Source: CAD feature listing. Evaluate the final solid. Frame: model axes, mm. Face numbers are marked on the shaded views. A direction names the side the tool comes from. Round coordinates to 2 decimals unless told otherwise and drop trailing zeros. Order: outer loops, then holes, each group sorted by start corner. A loop starts at its lowest first (then second) coordinate and runs counter-clockwise, first axis right, second up. Notation, with made-up numbers: (72, 41) -> (79, 41) arc R27 cw to (79, 59) -> close; hole circle Ø10 at (-37.75, 43.25). An arc over 180 degrees is marked (long way). Write item = value, one per line. Start each with the question number.
(1) Contact query for flat-ended pins moving along their axis: pin 1 Ø10.5 at (x, z) = (4, 6) entering from -Y; pin 2 Ø12 at (x, z) = (-2, -10) entering from +Y; pin 3 Ø5 at (y, z) = (-12, -2) entering from +X. Output: stop coordinate, or through.
(2) Cut plane C-C on z = -19. Return the cut outline in (x, y).
(3) Cut plane A-A on y = 0. Return the cut outline in (x, z), then the cut area to 3 significant figures.
(4) Draft query along Z for the marked faces 1, 2, 3 and 4. Return one class per face: released by +Z, released by -Z, zero draft, split by the parting line, or undercut.
(5) Cut plane D-D on x = 20.5. Return the cut outline in (y, z).
(6) Ray query, line 1 (Y direction, x = -0.5, z = -26.5); line 2 (X direction, y = 0, z = -26). Return the intervals inside material, ascending.
(7) Reachability of the marked faces 5, 6, 7, 8 and 9 from +Z, -Z, +X, -X, +Y, -Y: full face, straight path, thin tool, end or side. Return the list, or none.
from build123d import *

# Parameters (mm, degrees)
F2_W          = 60
F2_H          = 60
F3_DEPTH      = 30
F3_DEPTH_BACK = 30
F9_R          = 22.5
F10_DEPTH     = 12.5
F6_R          = 22.5
F11_DEPTH     = 12.5
F5_R          = 22.5
F12_DEPTH     = 12.5
F8_R          = 22.5
F13_DEPTH     = 12.5
F7_R          = 22.5
F14_DEPTH     = 12.5
F4_R          = 22.5
F15_DEPTH     = 12.5


with BuildPart() as f3:
    # F2 (on Top) → F3 (new body, two sides)
    with BuildSketch(Plane.XY) as f3_sk:
        Rectangle(F2_W, F2_H)
    extrude(amount=F3_DEPTH)
    extrude(f3_sk.sketch, amount=-F3_DEPTH_BACK)

    # F9 (on face) → F10 (cut)
    with BuildSketch(Plane(origin=(0, 0, -30), x_dir=(1, 0, 0), z_dir=(0, 0, -1))):
        Circle(F9_R)
    extrude(amount=-F10_DEPTH, mode=Mode.SUBTRACT)

    # F6 (on face) → F11 (cut)
    with BuildSketch(Plane(origin=(-30, 0, 0), x_dir=(0, -1, 0), z_dir=(-1, 0, 0))):
        Circle(F6_R)
    extrude(amount=-F11_DEPTH, mode=Mode.SUBTRACT)

    # F5 (on face) → F12 (cut)
    with BuildSketch(Plane.XZ.offset(30)):
        Circle(F5_R)
    extrude(amount=-F12_DEPTH, mode=Mode.SUBTRACT)

    # F8 (on face) → F13 (cut)
    with BuildSketch(Plane.YZ.offset(30)):
        Circle(F8_R)
    extrude(amount=-F13_DEPTH, mode=Mode.SUBTRACT)

    # F7 (on face) → F14 (cut)
    with BuildSketch(Plane(origin=(0, 30, 0), x_dir=(-1, 0, 0), z_dir=(0, 1, 0))):
        Circle(F7_R)
    extrude(amount=-F14_DEPTH, mode=Mode.SUBTRACT)

    # F4 (on face) → F15 (cut)
    with BuildSketch(Plane.XY.offset(30)):
        Circle(F4_R)
    extrude(amount=-F15_DEPTH, mode=Mode.SUBTRACT)


solid = f3.part
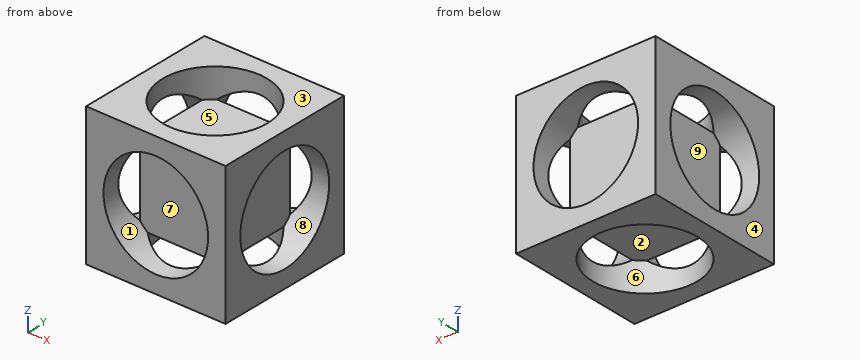
Evaluation:
q1.pin_1 = -17.5
q1.pin_2 = 17.5
q1.pin_3 = 17.5
q2.outline = (-30, -30) -> (-12.05, -30) -> (-12.05, -19) arc R22.5 cw to (-19, -12.05) -> (-30, -12.05) -> close; (-30, 12.05) -> (-19, 12.05) arc R22.5 cw to (-12.05, 19) -> (-12.05, 30) -> (-30, 30) -> close; (12.05, -30) -> (30, -30) -> (30, -12.05) -> (19, -12.05) arc R22.5 cw to (12.05, -19) -> close; (12.05, 19) arc R22.5 cw to (19, 12.05) -> (30, 12.05) -> (30, 30) -> (12.05, 30) -> close
q3.outline = (-30, -30) -> (-22.5, -30) -> (-22.5, -22.5) -> (-30, -22.5) -> close; (-30, 22.5) -> (-22.5, 22.5) -> (-22.5, 30) -> (-30, 30) -> close; (-17.5, -17.5) -> (17.5, -17.5) -> (17.5, 17.5) -> (-17.5, 17.5) -> close; (22.5, -30) -> (30, -30) -> (30, -22.5) -> (22.5, -22.5) -> close; (22.5, 22.5) -> (30, 22.5) -> (30, 30) -> (22.5, 30) -> close
q3.area = 1,450 mm^2
q4.face_1 = undercut
q4.face_2 = released by -Z
q4.face_3 = released by +Z
q4.face_4 = zero draft
q5.outline = (-30, -30) -> (-9.27, -30) -> (-9.27, -20.5) arc R22.5 cw to (-20.5, -9.27) -> (-30, -9.27) -> close; (-30, 9.27) -> (-20.5, 9.27) arc R22.5 cw to (-9.27, 20.5) -> (-9.27, 30) -> (-30, 30) -> close; (9.27, -30) -> (30, -30) -> (30, -9.27) -> (20.5, -9.27) arc R22.5 cw to (9.27, -20.5) -> close; (9.27, 20.5) arc R22.5 cw to (20.5, 9.27) -> (30, 9.27) -> (30, 30) -> (9.27, 30) -> close
q6.line_1 = -30 to -22.49, 22.49 to 30
q6.line_2 = -30 to -22.5, 22.5 to 30
q7.face_5 = +Z
q7.face_6 = -Z
q7.face_7 = -Y
q7.face_8 = +X
q7.face_9 = -X
